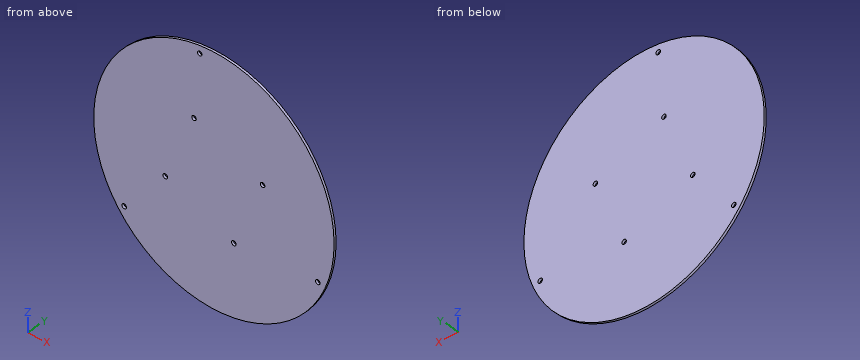
from build123d import *

# Parameters (mm, degrees)
CROQUIS1_R              = 160
CROQUIS1_R_2            = 3
SALIENTE_EXTRUIR2_DEPTH = 3


with BuildPart() as part:
    # Croquis1 → Saliente-Extruir2 (new body)
    with BuildSketch(Plane(origin=(0, 0, 0), x_dir=(1, 0, 0), z_dir=(0, 1, 0))):
        Circle(CROQUIS1_R)
        with Locations((138.31376779, 58.045685797)):
            Circle(CROQUIS1_R_2, mode=Mode.SUBTRACT)
        with Locations((-18.887845415, -148.806079498)):
            Circle(CROQUIS1_R_2, mode=Mode.SUBTRACT)
        with Locations((-64.794876894, 26.488184691)):
            Circle(CROQUIS1_R_2, mode=Mode.SUBTRACT)
        with Locations((26.488184691, 64.794876894)):
            Circle(CROQUIS1_R_2, mode=Mode.SUBTRACT)
        with Locations((64.794876894, -26.488184691)):
            Circle(CROQUIS1_R_2, mode=Mode.SUBTRACT)
        with Locations((-26.488184691, -64.794876894)):
            Circle(CROQUIS1_R_2, mode=Mode.SUBTRACT)
        with Locations((-119.425922375, 90.760393701)):
            Circle(CROQUIS1_R_2, mode=Mode.SUBTRACT)
    extrude(amount=SALIENTE_EXTRUIR2_DEPTH)


solid = part.part
Can you work these out from the model? Positions are in its coordinate system, mm. Round coordinates to 2 decimals unless told otherwise and drop trailing zeros. Order: outer loops, then holes, each group sorted by start corner. A loop starts at its lowest first (then second) coordinate and runs counter-clockwise, first axis right, second up. Notation, with made-up numbers: (11.25, 32) -> (42.25, 32) arc R5 cw to (42.25, 36) -> close; hole circle Ø10 at (20, 59.5). An arc over 180 degrees is marked (long way). Write each question's results on one line, items separated by ' | '. Start each with the question number.
Item 1: Please list where these lines run through material, in increasing order: L1, parallel to Z at x = 138.5, y = 2.75; L2, parallel to Z at x = -5, y = 1.75; L3, parallel to X at y = 2.25, z = 60.
Item 2: If we section it at B-B, the plane z = 40: Write out the boundary of the cut face in (x, y).
Item 3: If we section it at A-A, the plane y = 1.25: Write out the boundary of the cut face in (x, z), then the cut area to 3 significant figures.
Item 4: Will these pins go through, and if not, where does the flat tip stop? pin 1 (8 mm diameter, centred on x = -26.49, z = 64.79, fed in from +Y); pin 2 (1.5 mm diameter, centred on x = 26.5, y = 0.5, fed in from -Z); pin 3 (1.5 mm diameter, centred on y = 2.5, z = 56, fed in from -X).
Item 5: If we section it at C-C, the plane x = 34: Write out the boundary of the cut face in (y, z), then the cut area to 3 significant figures.
Results:
1) L1: z = -80.11 to -61.04, -55.05 to 80.11 | L2: z = -159.92 to 159.92 | L3: x = -148.32 to 148.32
2) outline: (-154.92, 0) -> (154.92, 0) -> (154.92, 3) -> (-154.92, 3) -> close
3) outline: circle Ø320 at (0, 0); hole circle Ø6 at (-119.43, -90.76); hole circle Ø6 at (-64.79, -26.49); hole circle Ø6 at (-26.49, 64.79); hole circle Ø6 at (-18.89, 148.81); hole circle Ø6 at (26.49, -64.79); hole circle Ø6 at (64.79, 26.49); hole circle Ø6 at (138.31, -58.05) | area: 80,200 mm2
4) pin 1: stops at y = 3 | pin 2: stops at z = -157.91 | pin 3: stops at x = -150.16
5) outline: (0, -156.35) -> (3, -156.35) -> (3, 156.35) -> (0, 156.35) -> close | area: 938 mm2
